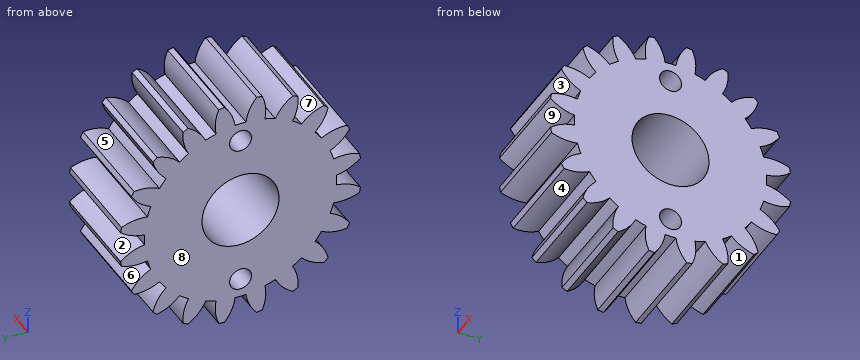
from build123d import *

# Parameters (mm, degrees)
BASPROSKE_W        = 9
BASPROSKE_H        = 11
TOOTHCUT_DEPTH     = 18.972200756
TEETHCUTS_COUNT    = 20
TEETHCUTS_ANGLE    = 342
BORSKE_R           = 3.5
BORE_DEPTH         = 50.0000508
SKETCH1_R          = 1
CUT_EXTRUDE1_DEPTH = 18.852389344


with BuildPart() as part:
    # BasProSke → Base-Revolve (revolve)
    with BuildSketch(Plane(origin=(0, 0, 0), x_dir=(1, 0, 0), z_dir=(0, 1, 0)), mode=Mode.PRIVATE) as base_revolve_sk:
        with Locations((4.5, 5.5)):
            Rectangle(BASPROSKE_W, BASPROSKE_H)
    revolve(base_revolve_sk.sketch.rotate(Axis((-10, 0, 0), (1, 0, 0)), 180), axis=Axis((-10, 0, 0), (1, 0, 0)))

    # TooCutSke → ToothCut (cut, through all)
    with BuildSketch(Plane(origin=(0, 0, 0), x_dir=(0, 0, -1), z_dir=(1, 0, 0))):
        with BuildLine():
            ThreePointArc((0.499924007, 8.734705318), (0, 8.749), (-0.499924007, 8.734705318))
            ThreePointArc((-0.499924007, 8.734705318), (-0.824302243, 9.905497836), (-1.485192705, 10.924909509))
            ThreePointArc((-1.485192705, 10.924909509), (0, 11.0254), (1.485192705, 10.924909509))
            ThreePointArc((1.485192705, 10.924909509), (0.824302243, 9.905497836), (0.499924007, 8.734705318))
        make_face()
    toothcut = extrude(amount=TOOTHCUT_DEPTH, mode=Mode.SUBTRACT)

    # TeethCuts: ToothCut ×20 about axis
    teethcuts_axis = Axis((-10, 0, 0), (1, 0, 0))
    for i in range(1, TEETHCUTS_COUNT):
        add(toothcut.rotate(teethcuts_axis, i * TEETHCUTS_ANGLE / (TEETHCUTS_COUNT - 1)), mode=Mode.SUBTRACT)

    # BorSke → Bore (cut, symmetric)
    with BuildSketch(Plane(origin=(0, 0, 0), x_dir=(0, 0, -1), z_dir=(1, 0, 0))):
        with Locations(Location((0, 0, 0), (0, 0, 180))):
            Circle(BORSKE_R)
    extrude(amount=BORE_DEPTH, both=True, mode=Mode.SUBTRACT)

    # Sketch1 → Cut-Extrude1 (cut, through all)
    with BuildSketch(Plane(origin=(9, 0, 0), x_dir=(0, 0, -1), z_dir=(1, 0, 0))):
        with Locations((-7, 0)):
            Circle(SKETCH1_R)
        with Locations((7, 0)):
            Circle(SKETCH1_R)
    extrude(amount=-CUT_EXTRUDE1_DEPTH, mode=Mode.SUBTRACT)


solid = part.part
Verification items for the finished model (mm, model axes). Face numbers are marked on the shaded views. A direction names the side the tool comes from. Give positions to 0.01 mm unless a question says otherwise; leave off trailing zeros. Order: outer loops, then holes, each group sorted by start corner. A loop starts at its lowest first (then second) coordinate and runs counter-clockwise, first axis right, second up. Notation, with made-up numbers: M 36,-20.75 L 63,-20.75 A38 cw 63,18.25 Z; hole C 41,74.5 d1. An arc over 180 degrees is marked long. Answer as a JSON object with one key per item and string values. Group by question number.
1) Cross-section at B-B (z = 2.75). Enter the section's corners in (x, y), then the cut area to 3 significant figures.
2) Cross-section at A-A (y = 0). Enter the section's corners in (x, z).
3) Cross-section at C-C (x = 4). Give the number of separate pieces and of enclosed holes in the cut face, then the cut area to 3 significant figures.
4) Cross-section at D-D (y = -4.25). Enter the section's corners in (x, z).
5) Access from +Z, -Z, +X, -X, +Y, -Y to the whole of each face (thin tool, end or side, straight path). Record for the marked faces 5, 6, 7, 8 and 9.
6) Depth check by flat-ended pin: pin 1 Ø1 at (x, z) = (8, 3) entering from +Y. Enter the tip coordinate at first touch or a pass-through.
7) Scan lines: line 1 along Y through (x, z) = (2.5, 0); line 2 along Z through (x, y) = (3, -9.5); line 3 along Y through (x, z) = (7, -7). Record each from-to range of solid material in increasing order. Write a range as [from, to].
8) Mould release check, pull along Y, two halves, no side actions. Record for the marked faces 1, 2, 3 and 4: released by +Y, released by -Y, zero draft, split by the parting line, or undercut.
Result sheet:
{
 "1": {"outline": "M 0,-8.31 L 9,-8.31 L 9,-2.17 L 0,-2.17 Z; M 0,2.17 L 9,2.17 L 9,8.31 L 0,8.31 Z", "area": "111 mm2"},
 "2": {"outline": "M 0,-8.75 L 9,-8.75 L 9,-8 L 0,-8 Z; M 0,-6 L 9,-6 L 9,-3.5 L 0,-3.5 Z; M 0,3.5 L 9,3.5 L 9,6 L 0,6 Z; M 0,8 L 9,8 L 9,8.75 L 0,8.75 Z"},
 "3": {"separate pieces": "1", "enclosed holes": "3", "area": "258 mm2"},
 "4": {"outline": "M 0,-9.55 L 9,-9.55 L 9,9.55 L 0,9.55 Z"},
 "5": {"face 5": "+X, -X", "face 6": "+X, -X, +Y", "face 7": "+Z, +X, -X", "face 8": "+Z, -Z, -X, +Y, -Y", "face 9": "+X, -X, -Y"},
 "6": {"pin 1": "stops at y = 8.73"},
 "7": {"line 1": "y = [-8.75, -3.5], [3.5, 8.75]", "line 2": "z = [-5.24, -4.19], [-2.29, -0.67], [0.67, 2.29], [4.19, 5.24]", "line 3": "y = [-7.78, -5.77], [-5.25, -1], [1, 5.25], [5.77, 7.78]"},
 "8": {"face 1": "undercut", "face 2": "released by +Y", "face 3": "released by -Y", "face 4": "undercut"}
}
